from build123d import *

# Parameters (mm, degrees)
BOSS_EXTRUDE1_DEPTH = 20
SKETCH2_R           = 1.5
CUT_EXTRUDE1_DEPTH  = 60
SKETCH4_R           = 2.5
BOSS_EXTRUDE2_DEPTH = 10
SKETCH5_R           = 3.5
BOSS_EXTRUDE3_DEPTH = 5
SKETCH6_R           = 1.25
CUT_EXTRUDE3_DEPTH  = 4
SKETCH7_W           = 20
SKETCH7_H           = 9.5
BOSS_EXTRUDE4_DEPTH = 8
SKETCH8_W           = 20
SKETCH8_H           = 9.5
BOSS_EXTRUDE5_DEPTH = 8
SKETCH9_R           = 1.5
CUT_EXTRUDE4_DEPTH  = 10


with BuildPart() as part:
    # Sketch1 → Boss-Extrude1 (new body)
    with BuildSketch(Plane.XY):
        Polygon((-14.5, 2.6), (-7.7, 2.6), (-7.7, 5), (-6.767766953, 5), (-4.4, 2.632233047), (-4.4, -2.632233047), (-6.767766953, -5), (-7.7, -5), (-7.7, -2.6), (-10.5, -2.6), (-10.5, -10.5), (30.5, -10.5), (30.5, -2.6), (27.7, -2.6), (27.7, -5), (26.767766953, -5), (24.4, -2.632233047), (24.4, 2.632233047), (26.767766953, 5), (27.7, 5), (27.7, 2.6), (34.5, 2.6), (34.5, -14.5), (15, -14.5), (15, -55), (5, -55), (5, -14.5), (-14.5, -14.5), align=None)
    extrude(amount=BOSS_EXTRUDE1_DEPTH)

    # Sketch2 → Cut-Extrude1 (cut)
    with BuildSketch(Plane.ZY.offset(14.5)):
        with Locations(Location((5, 0, 0), (0, 0, 270))):
            Circle(SKETCH2_R)
    extrude(amount=-CUT_EXTRUDE1_DEPTH, mode=Mode.SUBTRACT)

    # Sketch4 → Boss-Extrude2 (add)
    with BuildSketch(Plane.XY.offset(20)):
        with Locations((10, -49)):
            Circle(SKETCH4_R)
    extrude(amount=BOSS_EXTRUDE2_DEPTH)

    # Sketch5 → Boss-Extrude3 (add)
    with BuildSketch(Plane.XY.offset(20)):
        with Locations((10, -49)):
            Circle(SKETCH5_R)
    extrude(amount=BOSS_EXTRUDE3_DEPTH)

    # Sketch6 → Cut-Extrude3 (cut)
    with BuildSketch(Plane.XY.offset(30)):
        with Locations((10, -49)):
            Circle(SKETCH6_R)
    extrude(amount=-CUT_EXTRUDE3_DEPTH, mode=Mode.SUBTRACT)

    # Sketch7 → Boss-Extrude4 (add)
    with BuildSketch(Plane.ZY.offset(14.5)):
        with Locations((10, -9.75)):
            Rectangle(SKETCH7_W, SKETCH7_H)
    extrude(amount=BOSS_EXTRUDE4_DEPTH)

    # Sketch8 → Boss-Extrude5 (add)
    with BuildSketch(Plane(origin=(34.5, 0, 0), x_dir=(0, 0, -1), z_dir=(1, 0, 0))):
        with Locations((-10, -9.75)):
            Rectangle(SKETCH8_W, SKETCH8_H)
    extrude(amount=BOSS_EXTRUDE5_DEPTH)

    # Sketch9 → Cut-Extrude4 (cut)
    with BuildSketch(Plane.XY.offset(20)):
        with Locations((-17.5, -9.5)):
            Circle(SKETCH9_R)
        with Locations((37.5, -9.5)):
            Circle(SKETCH9_R)
    extrude(amount=-CUT_EXTRUDE4_DEPTH, mode=Mode.SUBTRACT)


solid = part.part
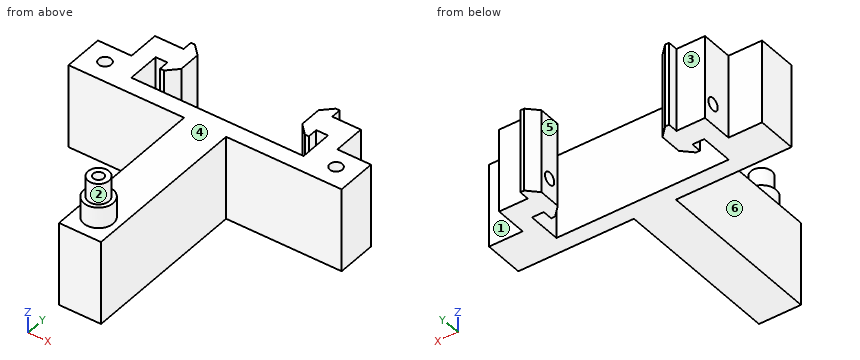
Design review of the part built by this model. Coordinates are the model's own, in mm. Face numbers are marked on the shaded views. A direction names the side the tool comes from. Round coordinates to 2 decimals unless told otherwise and drop trailing zeros. Order: outer loops, then holes, each group sorted by start corner. A loop starts at its lowest first (then second) coordinate and runs counter-clockwise, first axis right, second up.
1) Consider section B-B (y = -9.5). State the section outline as (x, z) points.
The answers:
outline: (-22.5, 0) - (-10.5, 0) - (-10.5, 20) - (-16, 20) - (-16, 10) - (-19, 10) - (-19, 20) - (-22.5, 20) - close; (30.5, 0) - (42.5, 0) - (42.5, 20) - (39, 20) - (39, 10) - (36, 10) - (36, 20) - (30.5, 20) - close
2) Clearance check with flat-ended pins moving along their axes: pin 1 Ø4 at (y, z) = (-29.5, 7) entering from +X; pin 2 Ø2.5 at (y, z) = (0.5, 11.5) entering from +X; pin 3 Ø0.9 at (x, y) = (-17.5, -10) entering from +Z. State where each tip first meets the part, or that it passes through.
The answers:
pin 1: stops at x = 15
pin 2: stops at x = 34.5
pin 3: stops at z = 10
3) Consider section C-C (x = 10). State the section outline as (y, z) points.
The answers:
outline: (-55, 0) - (-10.5, 0) - (-10.5, 20) - (-45.5, 20) - (-45.5, 25) - (-46.5, 25) - (-46.5, 30) - (-47.75, 30) - (-47.75, 26) - (-50.25, 26) - (-50.25, 30) - (-51.5, 30) - (-51.5, 25) - (-52.5, 25) - (-52.5, 20) - (-55, 20) - close
4) Draft analysis for pull direction X (two halves, no side actions). For the marked faces 4, 5 and 6, state which applies: released by +X, released by -X, zero draft, split by the parting line, or undercut.
The answers:
face 4: zero draft
face 5: undercut
face 6: released by -X
5) For L1, parallel to Y at x = 37.5, z = 17.75; L2, parallel to Y at x = 28.5, z = 8.5; L3, parallel to X at y = -3, z = 10, list the stretches that pass through material, from the lowest coordinate up.
The answers:
L1: y = -14.5 to -11, -8 to -5
L2: y = -14.5 to -10.5, -2.6 to 2.6
L3: x = -14.5 to -10.5, -7.7 to -4.77, 24.77 to 27.7, 30.5 to 34.5
6) Machinability: for the marked faces 1, 2 and 3, which of the approach directions +Z, -Z, +X, -X, +Y, -Y give a long, thin tool a straight path to every point of the face, cutting with its end or side? Answer none if there is none.
The answers:
face 1: +Z, -Z, +X, +Y
face 2: +Z
face 3: +Z, -Z, -X, +Y
7) Consider section D-D (y = 0). State the section outline as (x, z) points, plus the area to 3 significant figures.
The answers:
outline: (-14.5, 0) - (-4.4, 0) - (-4.4, 3.5) - (-14.5, 3.5) - close; (-14.5, 6.5) - (-4.4, 6.5) - (-4.4, 20) - (-14.5, 20) - close; (24.4, 0) - (34.5, 0) - (34.5, 3.5) - (24.4, 3.5) - close; (24.4, 6.5) - (34.5, 6.5) - (34.5, 20) - (24.4, 20) - close
area: 343 mm2
8) Consider section A-A (z = 11.75). Count the separate pieces of the cut face and the enclosed holes in it, plus the area to 3 significant figures.
The answers:
separate pieces: 1
enclosed holes: 2
area: 928 mm2
